Verification items for the finished model (mm, model axes). Face numbers are marked on the shaded views. A direction names the side the tool comes from. Coordinates: 2 decimals unless noted, no trailing zeros. Order: outer loops, then holes, each group sorted by start corner. A loop starts at its lowest first (then second) coordinate and runs counter-clockwise, first axis right, second up. Notation, with made-up numbers: (58, 77.25) -> (114, 77.25) arc R26 ccw to (114, 96.25) -> close; hole circle Ø9 at (83.5, 4.25). An arc over 180 degrees is marked (long way). Write item = value, one per line. Start each with the question number.
1. Cross-section at A-A on z = 0. Record the cut outline in (x, y).
2. Thickness scan on line 1 along Y through (x, z) = (2, -1); line 2 along Z through (x, y) = (-0.5, -21.5); line 3 along Z through (x, y) = (0, -72). Record the ranges inside material, lowest first. Write a range as from..to.
3. Go/stop test with flat-tipped pins: P1, Ø2, axis at x = 5.5, y = -11.5, coming from the +Z side; P2, Ø8, axis at y = -65.5, z = -5.5, coming from the -X side; P3, Ø8, axis at x = -10, y = -65, coming from the +Z side. Record where each tip stops, or that it passes through.
4. Set-up check for the marked faces 5 and 6: record each of +Z, -Z, +X, -X, +Y, -Y from which the full face is reachable in a straight line by a thin tool's end or side.
5. Release check for a two-part mould opening along X. For the marked faces 1, 2, 3 and 4 record: +X half, -X half, draft (parallel to the pull), parting line (faces both ways), or undercut.
6. Cross-section at B-B on x = 7. Record the cut outline in (y, z), plus the area to 3 significant figures.
7. Cross-section at D-D on x = 14.5. Record the cut outline in (y, z).
8. Cross-section at C-C on y = -18. Record the cut outline in (x, z).
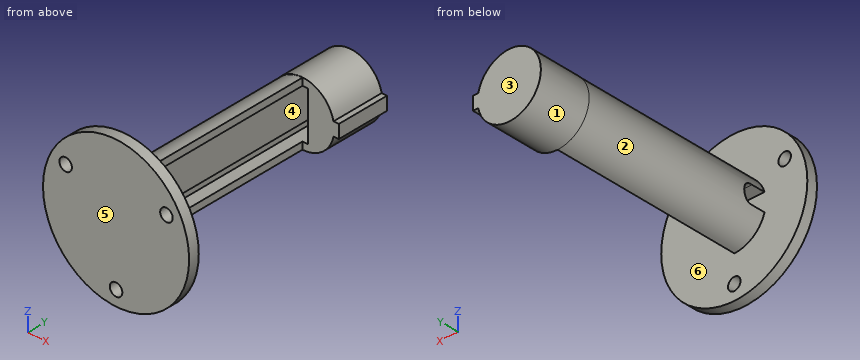
from build123d import *

# Parameters (mm, degrees)
PAD_DEPTH          = 15
POCKET_DEPTH       = 13
PAD001_DEPTH       = 55
POCKET001_DEPTH    = 7.601
SKETCH004_R        = 21
PAD002_DEPTH       = 3
SKETCH005_R        = 1.8
POCKET002_DEPTH    = 261.224272
POLARPATTERN_COUNT = 3


with BuildPart() as part:
    # Sketch → Pad (new body)
    with BuildSketch(Plane.XZ):
        with BuildLine():
            ThreePointArc((8.889624, 1.945402), (-9.099882, -0.046426), (8.90901, -1.854598))
            Line((10.40901, -1.854598), (8.90901, -1.854598))
            Line((10.40901, 1.945402), (10.40901, -1.854598))
            Line((8.889624, 1.945402), (10.40901, 1.945402))
        make_face()
    extrude(amount=PAD_DEPTH)

    # Sketch001 (on Face6 of Pad) → Pocket (cut)
    with BuildSketch(Plane.XZ.offset(15)):
        Polygon((-1.5, 7), (1.5, 7), (1.5, -7), (-3.348355, -7), (-3.348355, -3.808815), (-1.5, -3.808815), align=None)
    extrude(amount=-POCKET_DEPTH, mode=Mode.SUBTRACT)

    # Sketch002 (on Face5 of Pocket) → Pad001 (join)
    with BuildSketch(Plane.XZ.offset(15)):
        with BuildLine():
            Line((0, 7), (-1.5, 7))
            Line((-1.5, 7), (-1.5, -3.808815))
            Line((-1.5, -3.808815), (-3.348355, -3.808815))
            Line((-3.348355, -3.808815), (-3.348355, -7))
            Line((-3.348355, -7), (0, -7))
            Line((0, -7), (0, -9.054887))
            ThreePointArc((0, 9.054887), (-9.054887, 0), (0, -9.054887))
            Line((0, 7), (0, 9.054887))
        make_face()
    extrude(amount=PAD001_DEPTH)

    # Sketch003 (on Face19 of Pad001) → Pocket001 (cut, through all)
    with BuildSketch(Plane(origin=(-1.5, 0, 0), x_dir=(0, 0, 1), z_dir=(1, 0, 0))):
        with BuildLine():
            Line((-2.546247, 70), (-2.546247, 65.982418))
            ThreePointArc((-2.546247, 65.982418), (0.071035, 63.295116), (2.534594, 66.124008))
            Line((2.534594, 70), (2.534594, 66.124008))
            Line((-2.546247, 70), (2.534594, 70))
        make_face()
    extrude(amount=-POCKET001_DEPTH, mode=Mode.SUBTRACT)

    # Sketch004 (on Face14 of Pocket001) → Pad002 (join)
    with BuildSketch(Plane.XZ.offset(70)):
        Circle(SKETCH004_R)
    extrude(amount=PAD002_DEPTH)

    # Sketch005 (on Face3 of Pad002) → Pocket002 (cut, through all)
    with BuildSketch(Plane.XZ.offset(73)):
        with Locations((0, -16.72)):
            Circle(SKETCH005_R)
    pocket002 = extrude(amount=-POCKET002_DEPTH, mode=Mode.SUBTRACT)

    # PolarPattern: Pocket002 ×3 about axis
    polarpattern_axis = Axis((0, -73, 0), (0, -1, 0))
    for i in range(1, POLARPATTERN_COUNT):
        add(pocket002.rotate(polarpattern_axis, i * 360 / POLARPATTERN_COUNT), mode=Mode.SUBTRACT)


solid = part.part
Worked out:
q1.outline = (-21, -73) -> (21, -73) -> (21, -70) -> (-21, -70) -> close; (-9.1, -15) -> (-9.05, -15) -> (-9.05, -63.29) -> (-1.5, -63.29) -> (-1.5, -2) -> (1.5, -2) -> (1.5, -15) -> (10.41, -15) -> (10.41, 0) -> (-9.1, 0) -> close
q2.line_1 = -73..-70, -15..0
q2.line_2 = -9.04..-7, 7..9.04
q2.line_3 = -21..-18.52, -14.92..21
q3.P1 = 7.91
q3.P2 = -8.88
q3.P3 = 6.78
q4.face_5 = +Z, -Z, +X, -X, -Y
q4.face_6 = none
q5.face_1 = parting line
q5.face_2 = -X half
q5.face_3 = draft
q5.face_4 = undercut
q6.outline = (-73, -19.8) -> (-70, -19.8) -> (-70, 19.8) -> (-73, 19.8) -> close; (-15, -5.81) -> (0, -5.81) -> (0, 5.81) -> (-15, 5.81) -> close
q6.area = 293 mm²
q7.outline = (-73, -15.19) -> (-70, -15.19) -> (-70, 6.56) -> (-73, 6.56) -> close; (-73, 10.16) -> (-70, 10.16) -> (-70, 15.19) -> (-73, 15.19) -> close
q8.outline = (-3.35, -7) -> (-3.35, -3.81) -> (-1.5, -3.81) -> (-1.5, 7) -> (0, 7) -> (0, 9.05) arc R9.05 ccw to (0, -9.05) -> (0, -7) -> close
